Work out the finished part from the listing and answer in its coordinate system (mm). Give positions to 0.01 mm unless a question says otherwise; leave off trailing zeros. Loops run counter-clockwise (first coordinate to the right, second up) from the corner with the lowest first, then second, coordinate; pieces in that order, holes last. Notation, with made-up numbers: M 88,53.25 L 120,53.25 A18 cw 120,84.25 Z; hole C 37.5,88 d3. An arc over 180 degrees is marked long. Write item = value, one per line. Start each with the question number.
1. Section A-A on z = -102 is taken. Determine the outline of the cut face in (x, y), plus the area to 3 significant figures.
2. A flat-ended cylindrical pin translates along its axis: pin 1 Ø3 at (x, z) = (-178, 110) entering from +Y. Find the tip coordinate at first contact, or state that the pin passes through.
3. Consider L1, parallel to Z at x = 178, y = 2.2; L2, parallel to Z at x = 185, y = 2.9; L3, parallel to X at y = 2.25, z = -94. Determine where each line is inside the solid, lowest interval first. Write a range as [from, to].
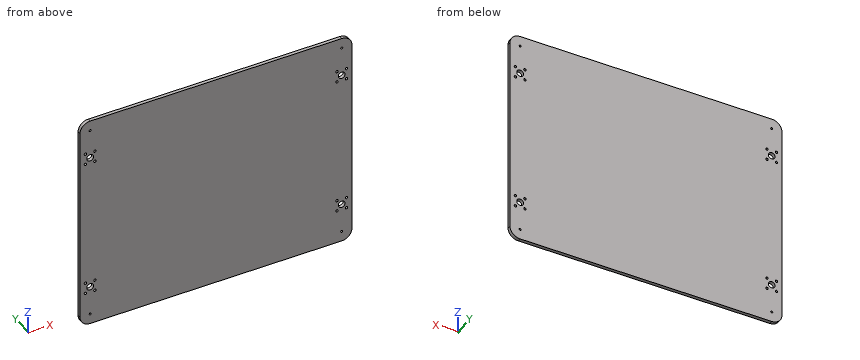
```python
from build123d import *

# Parameters (mm, degrees)
EXTRUDE_1_DEPTH                              = 5
FILLET_1_R                                   = 15
SKETCH_2_R                                   = 1.75
SKETCH_2_R_2                                 = 5
CUT_EXTRUDE_2_DEPTH                          = 257.173769149
MIRROR_1_AT_THE_SECOND_PLANE_COPY_1_SKET_R   = 1.75
MIRROR_1_AT_THE_SECOND_PLANE_COPY_1_SKET_R_2 = 5
MIRROR_1_AT_THE_SECOND_PLANE_COPY_1_DEPTH    = 257.173769149
SKETCH_3_R                                   = 1.5
CUT_EXTRUDE_3_DEPTH                          = 257.173769149
MIRROR_2_AT_THE_SECOND_PLANE_COPY_1_SKET_R   = 1.5
MIRROR_2_AT_THE_SECOND_PLANE_COPY_1_DEPTH    = 257.173769149


with BuildPart() as part:
    # 草图1 → 凸台-拉伸1 (new body)
    with BuildSketch(Plane(origin=(0, 0, 0), x_dir=(1, 0, 0), z_dir=(0, 1, 0))):
        Polygon((200, 0), (200, -160), (-200, -160), (-200, 0), (-200, 160), (200, 160), align=None)
    extrude(amount=EXTRUDE_1_DEPTH)

    # 圆角1
    fillet_1_edges = [part.edges().sort_by_distance(p)[0] for p in [
        (-200, 2.5, 160),
        (-200, 2.5, -160),
        (200, 2.5, -160),
        (200, 2.5, 160),
    ]]
    fillet(fillet_1_edges, radius=FILLET_1_R)

    # 草图2 → 切除-拉伸2 (cut, through all)
    with BuildSketch(Plane(origin=(0, 5, 0), x_dir=(1, 0, 0), z_dir=(0, 1, 0))):
        with Locations(Location((-192, 110, 0), (0, 0, 270))):
            Circle(SKETCH_2_R)
        with Locations(Location((-178, 110, 0), (0, 0, 270))):
            Circle(SKETCH_2_R)
        with Locations(Location((-178, 94, 0), (0, 0, 270))):
            Circle(SKETCH_2_R)
        with Locations(Location((-185, 102, 0), (0, 0, 270))):
            Circle(SKETCH_2_R_2)
        with Locations(Location((-192, 94, 0), (0, 0, 270))):
            Circle(SKETCH_2_R)
    cut_extrude_2 = extrude(amount=-CUT_EXTRUDE_2_DEPTH, mode=Mode.SUBTRACT)

    # 镜向1: 切除-拉伸2 across plane
    add(cut_extrude_2.mirror(Plane(origin=(0, 0, 0), x_dir=(0, 0, 1), z_dir=(1, 0, 0))), mode=Mode.SUBTRACT)

    # 镜向1 at the second plane: 切除-拉伸2 across plane
    add(cut_extrude_2.mirror(Plane.XY), mode=Mode.SUBTRACT)

    # 镜向1 at the second plane copy 1 sket → 镜向1 at the second plane copy 1 (cut, through all)
    with BuildSketch(Plane(origin=(0, 5, 0), x_dir=(-1, 0, 0), z_dir=(0, 1, 0))):
        with Locations(Location((-192, 110, 0), (0, 0, 270))):
            Circle(MIRROR_1_AT_THE_SECOND_PLANE_COPY_1_SKET_R)
        with Locations(Location((-178, 110, 0), (0, 0, 270))):
            Circle(MIRROR_1_AT_THE_SECOND_PLANE_COPY_1_SKET_R)
        with Locations(Location((-178, 94, 0), (0, 0, 270))):
            Circle(MIRROR_1_AT_THE_SECOND_PLANE_COPY_1_SKET_R)
        with Locations(Location((-185, 102, 0), (0, 0, 270))):
            Circle(MIRROR_1_AT_THE_SECOND_PLANE_COPY_1_SKET_R_2)
        with Locations(Location((-192, 94, 0), (0, 0, 270))):
            Circle(MIRROR_1_AT_THE_SECOND_PLANE_COPY_1_SKET_R)
    extrude(amount=-MIRROR_1_AT_THE_SECOND_PLANE_COPY_1_DEPTH, mode=Mode.SUBTRACT)

    # 草图3 → 切除-拉伸3 (cut, through all)
    with BuildSketch(Plane(origin=(0, 5, 0), x_dir=(1, 0, 0), z_dir=(0, 1, 0))):
        with Locations(Location((185, -145, 0), (0, 0, 270))):
            Circle(SKETCH_3_R)
    cut_extrude_3 = extrude(amount=-CUT_EXTRUDE_3_DEPTH, mode=Mode.SUBTRACT)

    # 镜向2: 切除-拉伸3 across plane
    add(cut_extrude_3.mirror(Plane.XY), mode=Mode.SUBTRACT)

    # 镜向2 at the second plane: 切除-拉伸3 across plane
    add(cut_extrude_3.mirror(Plane(origin=(0, 0, 0), x_dir=(0, 0, 1), z_dir=(1, 0, 0))), mode=Mode.SUBTRACT)

    # 镜向2 at the second plane copy 1 sket → 镜向2 at the second plane copy 1 (cut, through all)
    with BuildSketch(Plane(origin=(0, 5, 0), x_dir=(-1, 0, 0), z_dir=(0, 1, 0))):
        with Locations(Location((185, -145, 0), (0, 0, 270))):
            Circle(MIRROR_2_AT_THE_SECOND_PLANE_COPY_1_SKET_R)
    extrude(amount=-MIRROR_2_AT_THE_SECOND_PLANE_COPY_1_DEPTH, mode=Mode.SUBTRACT)


solid = part.part
```
Verdict:
q1.outline = M -200,0 L -190,0 L -190,5 L -200,5 Z; M -180,0 L 180,0 L 180,5 L -180,5 Z; M 190,0 L 200,0 L 200,5 L 190,5 Z
q1.area = 1,900 mm2
q2.pin_1 = through
q3.L1 = [-160, -111.75], [-108.25, -95.75], [-92.25, 92.25], [95.75, 108.25], [111.75, 160]
q3.L2 = [-160, -146.5], [-143.5, -107], [-97, 97], [107, 143.5], [146.5, 160]
q3.L3 = [-200, -193.75], [-190.25, -179.75], [-176.25, 176.25], [179.75, 190.25], [193.75, 200]
